Build history of the part. All positions in model axes, mm. A direction names the side the tool comes from. Give positions to 0.01 mm unless a question says otherwise; leave off trailing zeros. Write each loop counter-clockwise with the first axis right and the second up, starting at its lowest first coordinate (ties: lowest second). Pieces come first, ordered by that corner, then holes. Notation, with made-up numbers: (77, 57) -> (93, 57) arc R20 ccw to (93, 85) -> close; hole circle Ø8 at (60, -20). An arc over 180 degrees is marked (long way). Write item = value, one per line. Start each with the question number.
Q1. Saw through at D-D, the plane x = -1.5. List the corners of the cut face in (y, z).
Q2. Wall check: line 1 (Y direction, x = -21, z = 8.75); line 2 (Z direction, x = -18.5, y = -6). Give the ranges that are in metal, low to high.
Q3. Saw through at A-A, the plane z = 0. List the corners of the cut face in (x, y).
Q4. Saw through at B-B, the plane x = -17. List the corners of the cut face in (y, z), then the cut area to 3 significant figures.
Q5. Drop flat-ended pins along their axis: P1, Ø14, axis at y = -12, z = 3, coming from the -X side; P2, Ø6.5, axis at y = 16.5, z = 0.5, coming from the -X side; P3, Ø1, axis at y = -18.5, z = 1, coming from the +X side; P4, Ø12, axis at y = -5.5, z = 5, coming from the +X side. Give the stop position or say it passes through.
Q6. Mould opens along Z. For faces 4 (the face through (-16, 0, -11.938)), 5 (the face through (-2.175, -18.618, 9.794)), 6 (the face through (-21.159, 15.853, 9.105)), 7 (the face through (-13.07, -6.2, 1.38)) say: pulls with the +Z half, pulls with the -Z half, needs draft (parallel to the pull), parting line crosses it, or undercut.
Q7. Saw through at C-C, the plane y = -5.5. List the corners of the cut face in (x, z).
Q8. Tool access for faces 1 (the face through (-11, 13.081, 0)), 2 (the face through (-12, 24.003, 0)), 3 (the face through (-20, 0, -6.35)): list every direction of +Z, -Z, +X, -X, +Y, -Y with a clear straight run to the whole face (end or side of a thin tool).
from build123d import *

# Parameters (mm, degrees)
SKETCH1_R               = 10.033
BOSS_EXTRUDE1_DEPTH     = 24.003
SKETCH3_R               = 2.54
SKETCH3_W               = 24.13
SKETCH3_H               = 26.162
CUT_EXTRUDE1_DEPTH      = 12.938
CUT_EXTRUDE1_DEPTH_BACK = 12.938
SKETCH5_R               = 6.35
CUT_EXTRUDE2_DEPTH      = 26.908
FILLET1_R               = 5.08


with BuildPart() as part:
    # Sketch1 → Boss-Extrude1 (new body, symmetric)
    with BuildSketch(Plane(origin=(0, 0, 0), x_dir=(1, 0, 0), z_dir=(0, 1, 0))):
        with BuildLine():
            Line((0, 11.938), (-25.908, 11.938))
            Line((-25.908, 11.938), (-25.908, 6.35))
            Line((-25.908, 6.35), (-13.97, 6.35))
            Line((-13.97, 6.35), (-13.97, -6.35))
            Line((-13.97, -6.35), (-25.908, -6.35))
            Line((-25.908, -6.35), (-25.908, -11.938))
            Line((-25.908, -11.938), (0, -11.938))
            ThreePointArc((0, -11.938), (11.938, 0), (0, 11.938))
        make_face()
        Circle(SKETCH1_R, mode=Mode.SUBTRACT)
    extrude(amount=BOSS_EXTRUDE1_DEPTH, both=True)

    # Sketch3 → Cut-Extrude1 (cut, two sides)
    with BuildSketch(Plane.XY) as cut_extrude1_sk:
        with Locations((-20.828, 13.335)):
            Circle(SKETCH3_R)
        with Locations((-20.828, -13.335)):
            Circle(SKETCH3_R)
        with Locations((-0.127, 0)):
            Rectangle(SKETCH3_W, SKETCH3_H)
    extrude(amount=CUT_EXTRUDE1_DEPTH, mode=Mode.SUBTRACT)
    extrude(cut_extrude1_sk.sketch, amount=-CUT_EXTRUDE1_DEPTH_BACK, mode=Mode.SUBTRACT)

    # Sketch5 → Cut-Extrude2 (cut, through all)
    with BuildSketch(Plane(origin=(0, 0, 0), x_dir=(0, 0, -1), z_dir=(1, 0, 0))):
        Circle(SKETCH5_R)
    extrude(amount=-CUT_EXTRUDE2_DEPTH, mode=Mode.SUBTRACT)

    # Fillet1
    fillet1_edges = [part.edges().sort_by_distance(p)[0] for p in [
        (-25.908, 24.003, -9.144),
        (-25.908, 24.003, 9.144),
        (-25.908, -24.003, 9.144),
        (-25.908, -24.003, -9.144),
    ]]
    fillet(fillet1_edges, radius=FILLET1_R)


solid = part.part
Report:
q1.outline = (-24, -11.94) -> (-13.08, -11.94) -> (-13.08, -9.92) -> (-24, -9.92) -> close; (-24, 9.92) -> (-13.08, 9.92) -> (-13.08, 11.94) -> (-24, 11.94) -> close; (13.08, -11.94) -> (24, -11.94) -> (24, -9.92) -> (13.08, -9.92) -> close; (13.08, 9.92) -> (24, 9.92) -> (24, 11.94) -> (13.08, 11.94) -> close
q2.line_1 = -24 to -15.87, -10.8 to 10.8, 15.87 to 24
q2.line_2 = -11.94 to -6.35, 6.35 to 11.94
q3.outline = (-13.97, -24) -> (-10.03, -24) -> (-10.03, -13.08) -> (-12.19, -13.08) -> (-12.19, -6.35) -> (-13.97, -6.35) -> close; (-13.97, 6.35) -> (-12.19, 6.35) -> (-12.19, 13.08) -> (-10.03, 13.08) -> (-10.03, 24) -> (-13.97, 24) -> close; (10.03, -24) -> (11.94, -24) -> (11.94, -13.08) -> (10.03, -13.08) -> close; (10.03, 13.08) -> (11.94, 13.08) -> (11.94, 24) -> (10.03, 24) -> close
q4.outline = (-24, -11.94) -> (24, -11.94) -> (24, -6.35) -> (-24, -6.35) -> close; (-24, 6.35) -> (24, 6.35) -> (24, 11.94) -> (-24, 11.94) -> close
q4.area = 537 mm2
q5.P1 = -25.91
q5.P2 = -13.97
q5.P3 = 11.93
q5.P4 = -12.19
q6.face_4 = pulls with the -Z half
q6.face_5 = undercut
q6.face_6 = needs draft
q6.face_7 = undercut
q7.outline = (-25.91, -11.94) -> (-12.19, -11.94) -> (-12.19, -3.17) -> (-13.97, -3.17) -> (-13.97, -6.35) -> (-25.91, -6.35) -> close; (-25.91, 6.35) -> (-13.97, 6.35) -> (-13.97, 3.17) -> (-12.19, 3.17) -> (-12.19, 11.94) -> (-25.91, 11.94) -> close
q8.face_1 = +Z, -Z, +X
q8.face_2 = +Z, -Z, +X, -X, +Y
q8.face_3 = -X, +Y, -Y
